from build123d import *

# Parameters (mm, degrees)
F1_DEPTH = 304.8
F2_R     = 4.572


with BuildPart() as f1:
    # F0 (on Right) → F1 (new body, symmetric)
    with BuildSketch(Plane.YZ):
        Polygon((-493.39557, -659.903709), (268.60443, -659.903709), (268.60443, 457.696393), (65.40442, 457.696393), (-151.710834, 251.400065), (-493.39557, 152.896393), align=None)
    extrude(amount=F1_DEPTH, both=True)

    # F2
    f2_edges = [f1.edges().sort_by_distance(p)[0] for p in [
        (-304.8, 167.004425, 457.696393),
        (-304.8, 268.60443, -101.103658),
    ]]
    fillet(f2_edges, radius=F2_R)


solid = f1.part
Design review of the part built by this model. Coordinates are the model's own, in mm. Round coordinates to 2 decimals unless told otherwise and drop trailing zeros. Loops run counter-clockwise (first coordinate to the right, second up) from the corner with the lowest first, then second, coordinate; pieces in that order, holes last. Notation, with made-up numbers: (26, 3) -> (58, 3) arc R31 ccw to (58, 39) -> close; hole circle Ø2 at (-6, -39.5). An arc over 180 degrees is marked (long way). Use one line per item in the form item = value. Start each with the question number.
Q1. We need section A-A on x = -185.5. Give the boundary of the cut face in (y, z), then the cut area to 3 significant figures.
Q2. We need section B-B on z = 316.5. Give the boundary of the cut face in (x, y).
Q3. Wall thickness on line 1 along Z through (x, y) = (152, -69); line 2 along Z through (x, y) = (237, -151.5); line 3 along Y through (x, z) = (-17, 289): over which ranges is each line inside the solid? List them lowest first. Write a range as [from, to].
Q4. We need section C-C on y = -237. Give the boundary of the cut face in (x, z), then the cut area to 3 significant figures.
Q5. We need section D-D on y = 15.5. Give the boundary of the cut face in (x, z).
Calculated:
q1.outline = (-493.4, -659.9) -> (268.6, -659.9) -> (268.6, 457.7) -> (65.4, 457.7) -> (-151.71, 251.4) -> (-493.4, 152.9) -> close
q1.area = 742,000 mm²
q2.outline = (-304.8, -83.2) -> (304.8, -83.2) -> (304.8, 268.6) -> (-300.23, 268.6) arc R4.57 ccw to (-304.8, 264.03) -> close
q3.line_1 = [-659.9, 329.99]
q3.line_2 = [-659.9, 251.6]
q3.line_3 = [-112.14, 268.6]
q4.outline = (-304.8, -659.9) -> (304.8, -659.9) -> (304.8, 226.81) -> (-304.8, 226.81) -> close
q4.area = 541,000 mm²
q5.outline = (-304.8, -659.9) -> (304.8, -659.9) -> (304.8, 410.28) -> (-304.8, 410.28) -> close
